from build123d import *

# Parameters (mm, degrees)
EXTRUDE_1_DEPTH          = 96.5
CUT_EXTRUDE_1_DEPTH      = 97.93327602
CUT_EXTRUDE_1_DEPTH_BACK = 10
SKETCH_2_R               = 1.2
SKETCH_2_3_R             = 2.05
CUT_EXTRUDE_2_DEPTH      = 2
CHAMFER_3_SIZE           = 2
SKETCH_3_W               = 1.8
SKETCH_3_H               = 7.4
CUT_EXTRUDE_3_DEPTH      = 1.9
CHAMFER_4_SIZE           = 0.2
CHAMFER_5_SIZE           = 0.6
CHAMFER_2_SIZE           = 1
SKETCH_4_W               = 1.3
SKETCH_4_H               = 30
EXTRUDE_2_DEPTH          = 3
CHAMFER_6_SIZE           = 3
CHAMFER_1_SIZE           = 1
CHAMFER_7_SIZE           = 0.4


# Some blends are built 0.0001 mm under size
with BuildPart() as part:
    # 草图1 → 凸台-拉伸1 (new body)
    with BuildSketch(Plane.XY):
        Polygon((0, 0), (7, 0), (7, 4), (0, 4), (-1.8, 4), (-1.8, -1.9), (0, -1.9), align=None)
    extrude(amount=-EXTRUDE_1_DEPTH)

    # 草图2 → 切除-拉伸1 (cut, two sides: drawn at the far end of the back side and taken through both)
    with BuildSketch(Plane(origin=(0, 4, 0), x_dir=(1, 0, 0), z_dir=(0, 1, 0)).offset(-CUT_EXTRUDE_1_DEPTH_BACK)):
        with Locations(Location((4.2, 79.25, 0), (0, 0, 90))):
            Circle(SKETCH_2_R)
        with Locations(Location((4.2, 17.25, 0), (0, 0, 90))):
            Circle(SKETCH_2_R)
    extrude(amount=CUT_EXTRUDE_1_DEPTH + CUT_EXTRUDE_1_DEPTH_BACK, mode=Mode.SUBTRACT)

    # 草图2<3> → 切除-拉伸2 (cut)
    with BuildSketch(Plane(origin=(0, 4, 0), x_dir=(1, 0, 0), z_dir=(0, 1, 0))):
        with Locations(Location((4.2, 79.25, 0), (0, 0, 270))):
            Circle(SKETCH_2_3_R)
        with Locations(Location((4.2, 17.25, 0), (0, 0, 270))):
            Circle(SKETCH_2_3_R)
    extrude(amount=-CUT_EXTRUDE_2_DEPTH, mode=Mode.SUBTRACT)

    # 倒角3
    chamfer_3_edges = [part.edges().sort_by_distance(p)[0] for p in [
        (-1.8, 4, -48.25),
    ]]
    chamfer(chamfer_3_edges, length=CHAMFER_3_SIZE)

    # 草图3 → 切除-拉伸3 (cut)
    with BuildSketch(Plane.XZ.offset(1.9)):
        with Locations((-0.9, -92.8)):
            Rectangle(SKETCH_3_W, SKETCH_3_H)
        with Locations((-0.9, -3.7)):
            Rectangle(SKETCH_3_W, SKETCH_3_H)
    extrude(amount=-CUT_EXTRUDE_3_DEPTH, mode=Mode.SUBTRACT)

    # 倒角4
    chamfer_4_edges = [part.edges().sort_by_distance(p)[0] for p in [
        (-1.8, -1.9, -48.25),
        (0, -1.9, -48.25),
        (-1.8, -0.95, -89.1),
        (0, -0.95, -89.1),
        (-1.8, 0, -92.8),
        (-1.8, -0.95, -7.4),
        (0, -0.95, -7.4),
        (-1.8, 0, -3.7),
    ]]
    chamfer(chamfer_4_edges, length=CHAMFER_4_SIZE)

    # 倒角5
    # the kernel refuses this chamfer: 0.6 mm, written as the material it takes off along each edge
    with BuildSketch(Plane(origin=(1.343009793, -1.9, -89.1), x_dir=(0, 0.9996219169112965, -0.027495876610595982), z_dir=(-1, 0, 0))) as chamfer_5_piece_1:
        Polygon((CHAMFER_5_SIZE * 0.999621916911, -CHAMFER_5_SIZE * 0.0274958766106), (-CHAMFER_5_SIZE * 0.0274958766106, -CHAMFER_5_SIZE * 0.999621916911), (0, 0), align=None)
    extrude(amount=4.486019586, mode=Mode.SUBTRACT)
    with BuildSketch(Plane(origin=(1.343009793, -1.9, -7.4), x_dir=(0, 0.9996219169112968, 0.027495876610585925), z_dir=(-1, 0, 0))) as chamfer_5_piece_2:
        Polygon((CHAMFER_5_SIZE * 0.999621916911, CHAMFER_5_SIZE * 0.0274958766106), (-CHAMFER_5_SIZE * 0.0274958766106, CHAMFER_5_SIZE * 0.999621916911), (0, 0), align=None)
    extrude(amount=4.486019586, mode=Mode.SUBTRACT)

    # 倒角2
    # the kernel refuses this chamfer: 1 mm, written as the material it takes off along each edge
    with BuildSketch(Plane(origin=(7, 4, 2.571682988), x_dir=(-0.9996219169112968, 0.027495876610586487, 0), z_dir=(0, 0, -1))) as chamfer_2_piece_1:
        Polygon((CHAMFER_2_SIZE * 0.999621916911, -CHAMFER_2_SIZE * 0.0274958766106), (-CHAMFER_2_SIZE * 0.0274958766106, -CHAMFER_2_SIZE * 0.999621916911), (0, 0), align=None)
    extrude(amount=101.643365976, mode=Mode.SUBTRACT)

    # 草图4 → 凸台-拉伸2 (add)
    with BuildSketch(Plane(origin=(0, 0, 0), x_dir=(1, 0, 0), z_dir=(0, 1, 0))):
        with Locations((6.35, 48.25)):
            Rectangle(SKETCH_4_W, SKETCH_4_H)
    extrude(amount=-EXTRUDE_2_DEPTH)

    # 倒角6
    chamfer_6_edges = [part.edges().sort_by_distance(p)[0] for p in [
        (6.35, 0, -33.25),
        (6.35, 0, -63.25),
    ]]
    chamfer(chamfer_6_edges, length=CHAMFER_6_SIZE - 0.0001)  # a hair under: the kernel refuses the full size

    # 倒角1
    chamfer_1_edges = [part.edges().sort_by_distance(p)[0] for p in [
        (7, 0, -81.37495),
        (7, 0, -15.12505),
    ]]
    chamfer(chamfer_1_edges, length=CHAMFER_1_SIZE)

    # 倒角7
    chamfer_7_edges = [part.edges().sort_by_distance(p)[0] for p in [
        (5.7, -3, -48.25),
    ]]
    chamfer(chamfer_7_edges, length=CHAMFER_7_SIZE)


solid = part.part
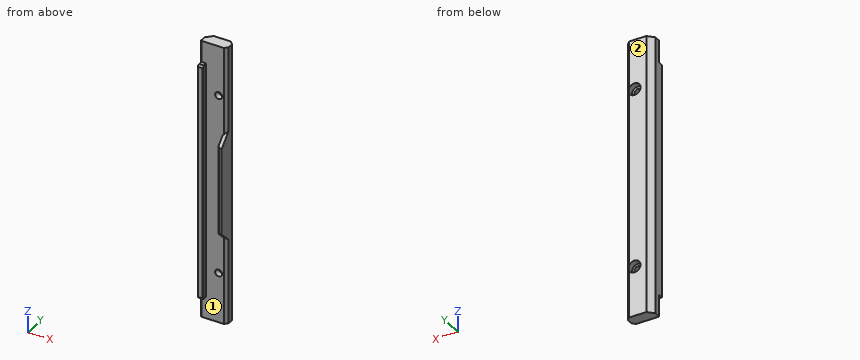
Verification items for the finished model (mm, model axes). Face numbers are marked on the shaded views. Round coordinates to 2 decimals unless told otherwise and drop trailing zeros. Order: outer loops, then holes, each group sorted by start corner. A loop starts at its lowest first (then second) coordinate and runs counter-clockwise, first axis right, second up.
1. Section check A-A on x = 4.2. Record the cut outline in (y, z), then the cut area to 3 significant figures.
Final values:
outline: (0, -96.5) - (4, -96.5) - (4, -81.3) - (2, -81.3) - (2, -80.45) - (0, -80.45) - close; (0, -78.05) - (2, -78.05) - (2, -77.2) - (4, -77.2) - (4, -19.3) - (2, -19.3) - (2, -18.45) - (0, -18.45) - close; (0, -16.05) - (2, -16.05) - (2, -15.2) - (4, -15.2) - (4, 0) - (0, 0) - close
area: 360 mm2
2. Section check B-B on z = -79.25. Record the cut outline in (x, y).
Final values:
outline: (-1.8, -1.7) - (-1.6, -1.9) - (-0.2, -1.9) - (0, -1.7) - (0, 0) - (3, 0) - (3, 2) - (2.15, 2) - (2.15, 4) - (0.2, 4) - (-1.8, 2) - close; (5.4, 0) - (6, 0) - (7, 1) - (7, 3) - (6.25, 3.75) - (6.25, 2) - (5.4, 2) - close
3. Go/stop test with flat-tipped pins: P1, Ø3, axis at x = 4.2, z = -79.25, coming from the +Y side; P2, Ø1.4, axis at x = 4.2, z = -17.25, coming from the +Y side; P3, Ø5, axis at x = 4, z = -68, coming from the -Y side; P4, Ø2.5, axis at x = 1.5, z = -38.5, coming from the -Y side. Record where each tip stops, or that it passes through.
Final values:
P1: stops at y = 2
P2: passes through
P3: stops at y = -0.08
P4: stops at y = 0
4. Thickness scan on L1, parallel to Z at x = 4.2, y = 2.9; L2, parallel to Z at x = 2.75, y = 3; L3, parallel to X at y = -1, z = -51.5. Record the ranges inside material, lowest first.
Final values:
L1: z = -96.5 to -81.3, -77.2 to -19.3, -15.2 to 0
L2: z = -96.5 to -80.7, -77.8 to -18.7, -15.8 to 0
L3: x = -1.8 to 0, 5.7 to 7
5. Release check for a two-part mould opening along X. For the marked faces 1 and 2 record: +X half, -X half, draft (parallel to the pull), parting line (faces both ways), or undercut.
Final values:
face 1: undercut
face 2: draft
6. Section check C-C on z = -69.5. Record the cut outline in (x, y), then the cut area to 3 significant figures.
Final values:
outline: (-1.8, -1.7) - (-1.6, -1.9) - (-0.2, -1.9) - (0, -1.7) - (0, 0) - (6, 0) - (7, 1) - (7, 3) - (6, 4) - (0.2, 4) - (-1.8, 2) - close
area: 35.6 mm2
